Here's the drawing with two shaded views (mm, measured from the low corner). I have some questions. A direction names the side the tool comes from. Coordinates: 2 decimals unless noted, no trailing zeros. Loops run counter-clockwise (first coordinate to the right, second up) from the corner with the lowest first, then second, coordinate; pieces in that order, holes last. Notation, with made-up numbers: M -10,49 L -5,49 A27 ccw -5,76 Z; hole C 55,62.25 d9. An arc over 180 degrees is marked long. Return JSON: item names as keys, results as strings. Group by question number.
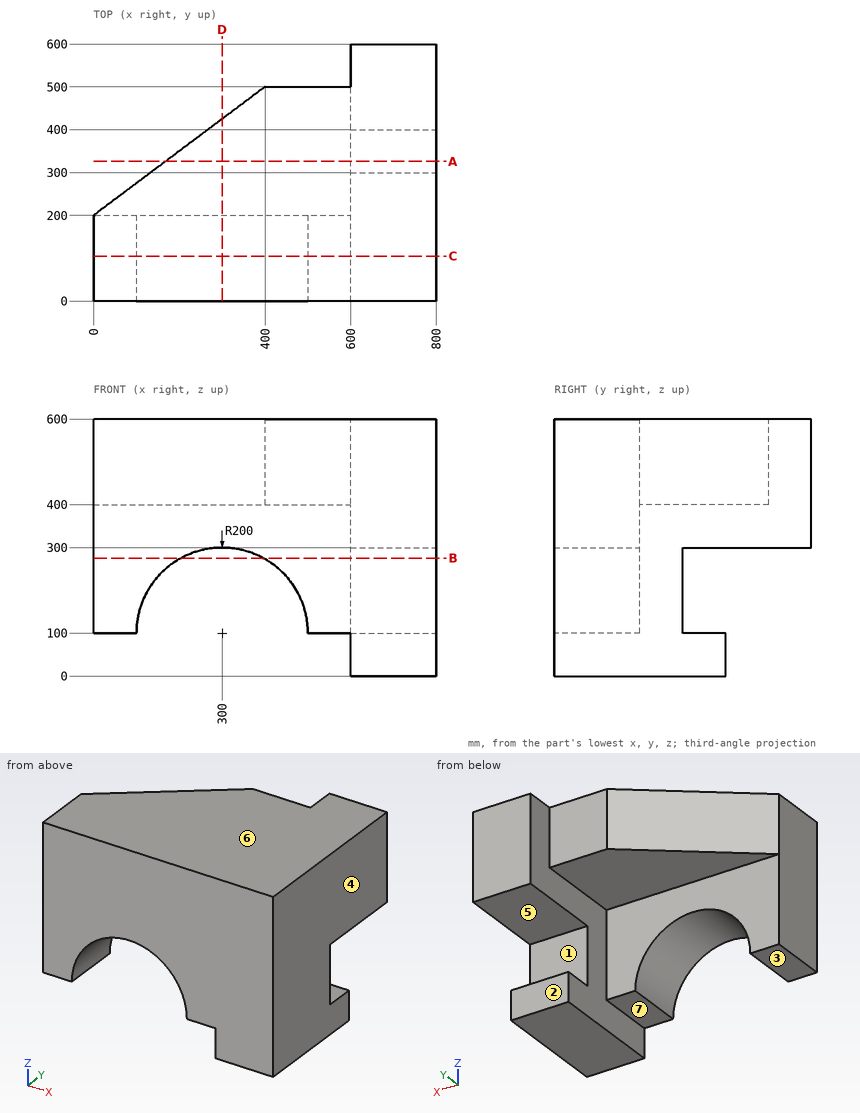
(1) Imagine slicing it at C-C, the plane y = 105. Write out the boundary of the cut face in (x, z).
(2) For the marked faces 1, 2 and 3, which set-ups out of +Z, -Z, +X, -X, +Y, -Y let a thin tool reach every point of the face, with its end or its side?
(3) Imagine slicing it at D-D, the plane x = 300. Write out the boundary of the cut face in (y, z).
(4) Imagine slicing it at B-B, the plane z = 275. Write out the boundary of the cut face in (x, y).
(5) Will these pins go through, and if not, where does the flat tip stop? P1, Ø1.5, axis at x = 370, y = 280, coming from the -Z side; P2, Ø1.5, axis at x = 303.5, z = 427.5, coming from the +Y side; P3, Ø2, axis at x = 150.5, z = 283, coming from the +Y side.
(6) We'd pull the mould along Z, two halves only. Please class the marked faces 4, 5, 6 and 7: +Z half, -Z half, draft (parallel to the pull), parting line (faces both ways), or undercut.
(7) If I drill on L1, parallel to Z at x = 723, y = 362; L2, parallel to Y at x = 187.5, z = 391; L3, parallel to Y at x = 507, z = 497, over which ranges is the centre line in solid material (lowest first)? Write a range as [from, to].
(8) Imagine slicing it at A-A, the plane y = 326. Write out the boundary of the cut face in (x, z), then the cut area to 3 significant figures.
Checks:
{
 "1": {"outline": "M 0,100 L 100,100 A200 cw 500,100 L 600,100 L 600,0 L 800,0 L 800,600 L 0,600 Z"},
 "2": {"face 1": "+X, -X, +Y", "face 2": "-Z, +X, -X, +Y", "face 3": "-Z, -X, +Y, -Y"},
 "3": {"outline": "M 0,300 L 200,300 L 200,400 L 425,400 L 425,600 L 0,600 Z"},
 "4": {"outline": "M 0,0 L 203.18,0 L 203.18,200 L 0,200 Z; M 396.82,0 L 800,0 L 800,300 L 600,300 L 600,200 L 396.82,200 Z"},
 "5": {"P1": "z = 400", "P2": "y = 428.19", "P3": "y = 200"},
 "6": {"face 4": "draft", "face 5": "undercut", "face 6": "+Z half", "face 7": "-Z half"},
 "7": {"L1": "[0, 100], [300, 600]", "L2": "[0, 200]", "L3": "[0, 500]"},
 "8": {"outline": "M 168,400 L 600,400 L 600,300 L 800,300 L 800,600 L 168,600 Z; M 600,0 L 800,0 L 800,100 L 600,100 Z", "area": "166,000 mm²"}
}
